Here's how the part is built. I have some questions about the finished solid (model axes, mm). A direction names the side the tool comes from. Coordinates: 2 decimals unless noted, no trailing zeros. Loops run counter-clockwise (first coordinate to the right, second up) from the corner with the lowest first, then second, coordinate; pieces in that order, holes last. Notation, with made-up numbers: M -10.75,-38.75 L 6.25,-38.75 A22 cw 6.25,-5.75 Z; hole C -35.75,43 d5. An arc over 180 degrees is marked long. Use one line per item in the form item = value. Start each with the question number.
(1) Imagine slicing it at A-A, the plane z = -43.5. Please give me the cut outline in (x, y).
(2) Thinking about a two-plate mould opening in X: for faces 3 (the flat face through (-202.5, 0, 3)), 4 (the flat face through (-3, 0, -200)), 5 (the flat face through (77.5, 0, 17)), which applies, +X half, -X half, draft (parallel to the pull), parting line (faces both ways), or undercut?
(3) Will these pins go through, and if not, where does the flat tip stop? P1, Ø3.5, axis at y = 0, z = 180, coming from the -X side; P2, Ø4, axis at y = 0, z = -180, coming from the -X side; P3, Ø2.5, axis at y = 0, z = -20, coming from the +X side.
(4) Please list where these lines run through material, in increasing order: L1, parallel to X at y = -4, z = 59.5; L2, parallel to Z at x = -194.5, y = 0; L3, parallel to Y at x = -62.5, z = -192.
(5) On a 3-axis mill with a long thin cutter (end or side, diameter ignored), from which of +Z, -Z, +X, -X, +Y, -Y can I reach the whole of each face in a straight line? I mean faces 1 (the flat face through (-3, -5, 3)), 2 (the flat face through (-42.5, 0, 23)). Say none if no direction works.
```python
from build123d import *

# Parameters (mm, degrees)
F1_DEPTH       = 5
F6_D           = 4.4
F6_DEPTH       = 12
F6_TIP         = 1.3218933619
F7_D           = 4.4
F7_DEPTH       = 12
F7_TIP         = 1.3218933619
F7_ON_F4_D     = 4.4
F7_ON_F4_DEPTH = 12
F7_ON_F4_TIP   = 1.3218933619
F7_ON_F5_D     = 4.4
F7_ON_F5_DEPTH = 12
F7_ON_F5_TIP   = 1.3218933619


# Not quite as in the source:
# - a feature names something its author has since deleted; it is built from what else it names


with BuildPart() as f1:
    # F0 (on Front) → F1 (new body, symmetric)
    with BuildSketch(Plane.XZ):
        Polygon((-202.5, -200), (202.5, -200), (202.5, 200), (87.5, 200), (87.5, -160), (77.5, -160), (77.5, 200), (-42.5, 200), (-42.5, -160), (-52.5, -160), (-52.5, 200), (-172.5, 200), (-172.5, -160), (-182.5, -160), (-182.5, 200), (-202.5, 200), align=None)
    extrude(amount=F1_DEPTH, both=True)

    # F6
    with Locations(Plane.XY.offset(200)):
        with Locations((0, 0)):
            Hole(F6_D / 2, depth=F6_DEPTH)
            with Locations((0, 0, -(F6_DEPTH + F6_TIP / 2))):  # 118° drill point
                Cone(0, F6_D / 2, F6_TIP, mode=Mode.SUBTRACT)

    # F7
    with Locations(Plane(origin=(-202.5, 0, 0), x_dir=(0, -1, 0), z_dir=(-1, 0, 0))):
        with Locations((0, -180), (0, -20), (0, 20), (0, 180)):
            Hole(F7_D / 2, depth=F7_DEPTH)
            with Locations((0, 0, -(F7_DEPTH + F7_TIP / 2))):  # 118° drill point
                Cone(0, F7_D / 2, F7_TIP, mode=Mode.SUBTRACT)

    # F7 on F4
    with Locations(Plane.YZ.offset(202.5)):
        with Locations((0, -180), (0, -20), (0, 180), (0, 20)):
            Hole(F7_ON_F4_D / 2, depth=F7_ON_F4_DEPTH)
            with Locations((0, 0, -(F7_ON_F4_DEPTH + F7_ON_F4_TIP / 2))):  # 118° drill point
                Cone(0, F7_ON_F4_D / 2, F7_ON_F4_TIP, mode=Mode.SUBTRACT)

    # F7 on F5
    with Locations(Plane(origin=(0, 0, -200), x_dir=(1, 0, 0), z_dir=(0, 0, -1))):
        with Locations((-182.5, 0), (-62.5, 0), (62.5, 0), (182.5, 0)):
            Hole(F7_ON_F5_D / 2, depth=F7_ON_F5_DEPTH)
            with Locations((0, 0, -(F7_ON_F5_DEPTH + F7_ON_F5_TIP / 2))):  # 118° drill point
                Cone(0, F7_ON_F5_D / 2, F7_ON_F5_TIP, mode=Mode.SUBTRACT)


solid = f1.part
```
Answer:
q1.outline = M -202.5,-5 L -182.5,-5 L -182.5,5 L -202.5,5 Z; M -172.5,-5 L -52.5,-5 L -52.5,5 L -172.5,5 Z; M -42.5,-5 L 77.5,-5 L 77.5,5 L -42.5,5 Z; M 87.5,-5 L 202.5,-5 L 202.5,5 L 87.5,5 Z
q2.face_3 = -X half
q2.face_4 = draft
q2.face_5 = undercut
q3.P1 = -190.23
q3.P2 = -190.38
q3.P3 = 189.93
q4.L1 = -202.5 to -182.5, -172.5 to -52.5, -42.5 to 77.5, 87.5 to 202.5
q4.L2 = -200 to -182.2, -177.8 to -22.2, -17.8 to 17.8, 22.2 to 177.8, 182.2 to 200
q4.L3 = -5 to -2.2, 2.2 to 5
q5.face_1 = +Z, -Z, +X, -X, -Y
q5.face_2 = +Z, +Y, -Y
